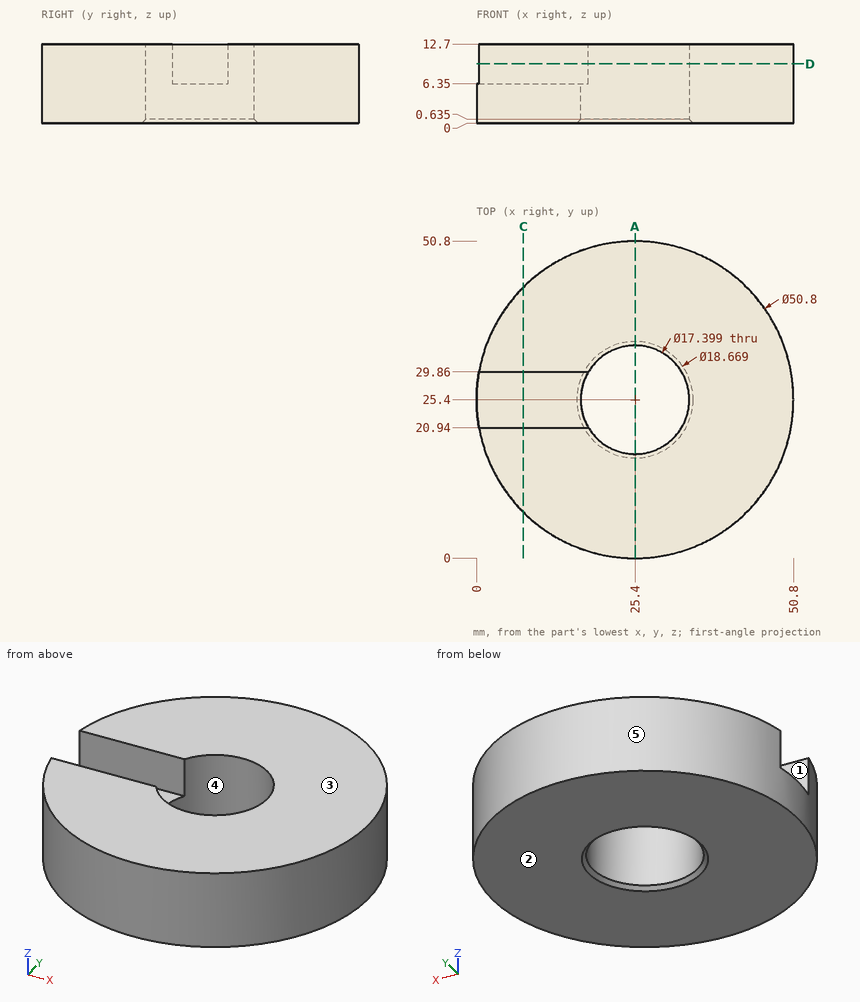
Drawing for the job (mm, zero at the part's lowest x, y, z). A direction names the side the tool comes from. Give positions to 0.01 mm unless a question says otherwise; leave off trailing zeros. Order: outer loops, then holes, each group sorted by start corner. A loop starts at its lowest first (then second) coordinate and runs counter-clockwise, first axis right, second up. Notation, with made-up numbers: M -35.5,-36.75 L 19.5,-36.75 A23 ccw 19.5,-6.75 Z; hole C -23,-35 d2. An arc over 180 degrees is marked long. Put each result on its own line as item: value. Start each with the question number.
(1) Drill centre lines: line 1 along Y through (x, z) = (25.4, 9); line 2 along X through (y, z) = (29, 1); line 3 along X through (y, z) = (25.4, 10.25). Where is each one in solid material? Low to high.
(2) Saw through at C-C, the plane x = 7.5. Write the cut outline in (y, z), then the cut area to 3 significant figures.
(3) Flat gauge pins, fed straight in: pin 1 Ø1.5 at (y, z) = (29, 3) entering from +X; pin 2 Ø1.9 at (x, z) = (8.5, 10.5) entering from -Y; pin 3 Ø5 at (x, z) = (14.5, 8) entering from -Y; pin 4 Ø1 at (x, y) = (32, 28.5) entering from +Z. Where does each tip first touch, or does it go through?
(4) Saw through at D-D, the plane z = 9.5. Write the cut outline in (x, y) (1 decimal), then the cut area to 3 significant figures.
(5) Mould opens along Y. For the marked faces 3, 4 and 5 say: +Y half, -Y half, draft (parallel to the pull), parting line (faces both ways), or undercut.
(6) Saw through at A-A, the plane x = 25.4. Write the cut outline in (y, z) (1 decimal).
(7) Which spindle directions (+Z, -Z, +X, -X, +Y, -Y) get a long thin tool onto all of the face, cutting with end or side? Do the marked faces 1 and 2. Say none if no direction does.
Check result:
1. line 1: y = 0 to 16.7, 34.1 to 50.8
1. line 2: x = 0.26 to 17.48, 33.32 to 50.54
1. line 3: x = 34.1 to 50.8
2. outline: M 7.38,0 L 43.42,0 L 43.42,12.7 L 29.86,12.7 L 29.86,6.35 L 20.94,6.35 L 20.94,12.7 L 7.38,12.7 Z
2. area: 401 mm2
3. pin 1: stops at x = 50.64
3. pin 2: stops at y = 5.63
3. pin 3: stops at y = 1.43
3. pin 4: passes through
4. outline: M 0.4,20.9 A25.4 ccw long 0.4,29.9 L 17.9,29.9 A8.7 cw long 17.9,20.9 Z
4. area: 1,640 mm2
5. face 3: draft
5. face 4: undercut
5. face 5: parting line
6. outline: M 0,0 L 16.1,0 L 16.7,0.6 L 16.7,12.7 L 0,12.7 Z; M 34.1,0.6 L 34.7,0 L 50.8,0 L 50.8,12.7 L 34.1,12.7 Z
7. face 1: +Z, -X
7. face 2: -Z, +X, -X, +Y, -Y
